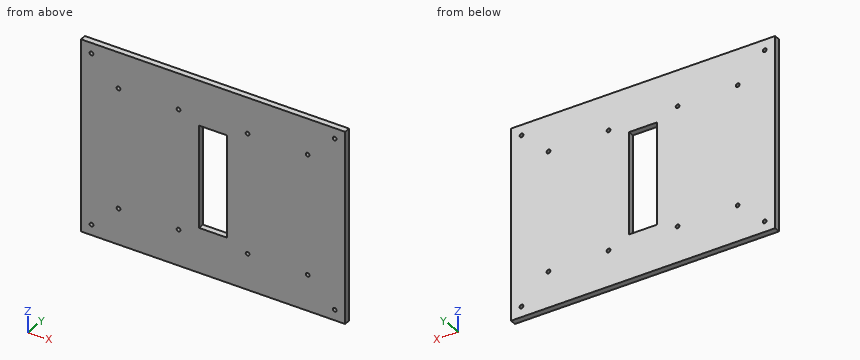
from build123d import *

# Parameters (mm, degrees)
SKETCH_1_W          = 176
SKETCH_1_H          = 128
EXTRUDE_1_DEPTH     = 4
SKETCH_3_W          = 18.73666899
SKETCH_3_H          = 68.153866922
CUT_EXTRUDE_2_DEPTH = 4
HOLE_WIZARD_M3_1_D  = 2.5


with BuildPart() as part:
    # 草图1 → 凸台-拉伸1 (new body)
    with BuildSketch(Plane(origin=(0, 0, 0), x_dir=(1, 0, 0), z_dir=(0, 1, 0))):
        with Locations((88, 64)):
            Rectangle(SKETCH_1_W, SKETCH_1_H)
    extrude(amount=EXTRUDE_1_DEPTH)

    # 草图3 → 切除-拉伸2 (cut)
    with BuildSketch(Plane(origin=(0, 4, 0), x_dir=(1, 0, 0), z_dir=(0, 1, 0))):
        with Locations((88, 64)):
            Rectangle(SKETCH_3_W, SKETCH_3_H)
    extrude(amount=-CUT_EXTRUDE_2_DEPTH, mode=Mode.SUBTRACT)

    # M3 螺纹孔1 (through all)
    with Locations(Plane(origin=(0, 4, 0), x_dir=(1, 0, 0), z_dir=(0, 1, 0))):
        with Locations((7, 121), (25, 104), (65, 104), (65, 24), (25, 24), (7, 7), (169, 7), (111, 24), (151, 24), (151, 104), (111, 104), (169, 121)):
            Hole(HOLE_WIZARD_M3_1_D / 2)


solid = part.part
Model file for the job. Use its own axes, mm. Give positions to 0.01 mm unless a question says otherwise; leave off trailing zeros. Order: outer loops, then holes, each group sorted by start corner. A loop starts at its lowest first (then second) coordinate and runs counter-clockwise, first axis right, second up. Notation, with made-up numbers: (13.5, -17.5) - (19.5, -17.5) arc R24 ccw to (19.5, 18.5) - close; hole circle Ø6 at (26, -36). An arc over 180 degrees is marked (long way). Return JSON: item names as keys, results as strings.
1) Cut at A-A, the plane z = -34. Give the cut face in (x, y), plus the area to 3 significant figures.
Geometry says:
{"outline": "(0, 0) - (78.63, 0) - (78.63, 4) - (0, 4) - close; (97.37, 0) - (176, 0) - (176, 4) - (97.37, 4) - close", "area": "629 mm²"}
2) Cut at C-C, the plane y = 1.95. Count the separate pieces of the cut face and the enclosed holes in it, plus the area to 3 significant figures.
Geometry says:
{"separate pieces": "1", "enclosed holes": "13", "area": "21,200 mm²"}
3) Cut at B-B, the plane x = 85.5. Give the cut face in (y, z).
Geometry says:
{"outline": "(0, -128) - (4, -128) - (4, -98.08) - (0, -98.08) - close; (0, -29.92) - (4, -29.92) - (4, 0) - (0, 0) - close"}
4) Probe line 1 (X direction, y = 1.8, z = -7); line 2 (Z direction, x = 169, y = 2.7); line 3 (Z direction, x = 111, y = 2.65). List the from-to ranges inside material, lowest first. Write a range as from..to.
Geometry says:
{"line 1": "0..5.75, 8.25..167.75, 170.25..176", "line 2": "-128..-122.25, -119.75..-8.25, -5.75..0", "line 3": "-128..-105.25, -102.75..-25.25, -22.75..0"}
5) Flat gauge pin, fed straight in: P1, Ø1.5, axis at x = 151, z = -24, coming from the -Y side. Where does the tip first touch, or does it go through?
Geometry says:
{"P1": "through"}
